Autodesk Inventor part; units mm, degrees
ref_plane "Work Plane1" through (0, 6, 0) normal (0, 1, 0) x (1, 0, 0)
ref_plane "Work Plane2" through (0, 7.6, 0) normal (0, 1, 0) x (1, 0, 0)
ref_plane "YZ Plane" through (0, 0, 0) normal (1, 0, 0) x (0, 1, 0)
sketch "Sketch1" plane through (0, 0, 0) normal (0, 1, 0) x (-1, 0, 0)
  circle A0 centre (0, 0) radius 1
  dimension "d0" = 2
extrude "Extrusion1" add sketch "Sketch1" along normal blind 6
chamfer "Chamfer1" distance 0.5 angle 45 1 edges at (1, 0, 0)
ref_plane "Work Plane1" through (0, 6, 0) normal (0, 1, 0) x (1, 0, 0)
sketch "Sketch2" plane through (0, 6, 0) normal (0, 1, 0) x (1, 0, 0)
  circle A0 centre (0, 0) radius 0.5
  circle A1 centre (0, 0) radius 1.5
  dimension "d7" = 3
extrude "Extrusion2" add sketch "Sketch2" along normal blind 1.6 contours A0 | A1
fillet "Fillet1" radius 0.5 1 edges at (-1.5, 7.6, 0)
ref_plane "Work Plane2" through (0, 7.6, 0) normal (0, 1, 0) x (1, 0, 0)
sketch "Sketch3" plane through (0, 7.6, 0) normal (0, 1, 0) x (1, 0, 0)
  line L0 (-0.75, 0.433) -> (0, 0.866)
  line L1 (0, 0.866) -> (0.75, 0.433)
  line L2 (0.75, 0.433) -> (0.75, -0.433)
  line L3 (0.75, -0.433) -> (0, -0.866)
  line L4 (0, -0.866) -> (-0.75, -0.433)
  line L5 (-0.75, -0.433) -> (-0.75, 0.433)
  point P0 (0, 0)
  point P1 (0, 0)
  dimension "d12" = 0.75
extrude "Extrusion3" cut sketch "Sketch3" against normal blind 1
thread "Thread1"
properties part number "M2x6mm_screw"
Can you work these out from the model? Positions are in its coordinate system, mm. A direction names the side the tool comes from. Round coordinates to 2 decimals unless told otherwise and drop trailing zeros. Order: outer loops, then holes, each group sorted by start corner. A loop starts at its lowest first (then second) coordinate and runs counter-clockwise, first axis right, second up. Notation, with made-up numbers: (-24, 75) - (29, 75) arc R19 cw to (29, 80) - close; hole circle Ø5 at (66.25, 64). An arc over 180 degrees is marked (long way). Answer in a Markdown table with one row per item.
(1) Which directions (+Z, -Z, +X, -X, +Y, -Y) give clear straight access to the entire face, cutting with the end or side of a thin tool? Please do faces 4 (the face through (0.75, 7, 0)), 5 (the face through (0, 3, 1)).
From the geometry:
| item | result |
|---|---|
| face 4 | +Y |
| face 5 | -Y |
(2) For P1, Ø1, axis at x = -0.5, y = 3, coming from the +Z side; P2, Ø1, axis at x = 0.5, z = -1, coming from the -Y side; P3, Ø0.8, axis at x = 0.5, z = 0.5, coming from the +Y side, each with a flat end and sliding along its axis, tell me the tip position at first contact or that it passes through.
From the geometry:
| item | result |
|---|---|
| P1 | stops at z = 1 |
| P2 | stops at y = 0.12 |
| P3 | stops at y = 7.6 |
(3) If we mould it in two halves opening along Z, with no side actions, what happens to faces 1 (the face through (-0.75, 7, 0)), 2 (the face through (0, 0, 0)), 3 (the face through (-1.5, 6.54, 0.07))? For each: released by +Z, released by -Z, zero draft, split by the parting line, or undercut.
From the geometry:
| item | result |
|---|---|
| face 1 | undercut |
| face 2 | zero draft |
| face 3 | split by the parting line |
(4) Please list where these lines run through material, in increasing order: L1, parallel to X at y = 6.5, z = -1.3; L2, parallel to Y at x = -0.1, z = 0; L3, parallel to Z at x = 0.4, y = 7. Write a range as from..to.
From the geometry:
| item | result |
|---|---|
| L1 | x = -0.75..0.75 |
| L2 | y = 0..6.6 |
| L3 | z = -1.45..-0.64, 0.64..1.45 |
(5) Suppose I cut it at B-B, the plane y = 6.25. Please give me the cut outline in (x, z).
From the geometry:
| item | result |
|---|---|
| outline | circle Ø3 at (0, 0) |
(6) Suppose I cut it at A-A, the plane z = 0. Please give me the cut outline in (x, y), plus the area to 3 significant figures.
From the geometry:
| item | result |
|---|---|
| outline | (-1.5, 6) - (-1, 6) - (-1, 0.5) - (-0.5, 0) - (0.5, 0) - (1, 0.5) - (1, 6) - (1.5, 6) - (1.5, 7.1) arc R0.5 ccw to (1, 7.6) - (0.75, 7.6) - (0.75, 6.6) - (-0.75, 6.6) - (-0.75, 7.6) - (-1, 7.6) arc R0.5 ccw to (-1.5, 7.1) - close |
| area | 14.9 mm2 |
